from build123d import *

# Parameters (mm, degrees)
F1_DEPTH = 50.8
F3_DEPTH = 25.4
F5_DEPTH = 25.4
F7_DEPTH = 2.54
F8_W     = 5.829871
F8_H     = 7.639144
F9_DEPTH = 2.54


with BuildPart() as f1:
    # F0 (on Front) → F1 (new body)
    with BuildSketch(Plane.XZ):
        Polygon((0, 6.35), (0, 0), (19.05, 0), (19.05, 63.5), (9.525, 63.5), (9.525, 6.35), align=None)
    extrude(amount=F1_DEPTH)

    # F2 (on face) → F3 (cut)
    with BuildSketch(Plane.XY.offset(6.35)):
        with BuildLine():
            ThreePointArc((0, -6.35), (1.859872, -1.859872), (6.35, 0))
            Line((6.35, 0), (0, 0))
            Line((0, 0), (0, -6.35))
        make_face()
        with BuildLine():
            Line((0, -50.8), (6.35, -50.8))
            ThreePointArc((6.35, -50.8), (1.859872, -48.940128), (0, -44.45))
            Line((0, -44.45), (0, -50.8))
        make_face()
    extrude(amount=-F3_DEPTH, mode=Mode.SUBTRACT)

    # F4 (on face) → F5 (cut)
    with BuildSketch(Plane(origin=(9.525, 0, 0), x_dir=(0, -1, 0), z_dir=(-1, 0, 0))):
        with BuildLine():
            ThreePointArc((0, 57.15), (1.859872, 61.640128), (6.35, 63.5))
            Line((6.35, 63.5), (0, 63.5))
            Line((0, 63.5), (0, 57.15))
        make_face()
        with BuildLine():
            ThreePointArc((44.45, 63.5), (48.940128, 61.640128), (50.8, 57.15))
            Line((50.8, 57.15), (50.8, 63.5))
            Line((50.8, 63.5), (44.45, 63.5))
        make_face()
    extrude(amount=-F5_DEPTH, mode=Mode.SUBTRACT)

    # F6 (on face) → F7 (cut)
    with BuildSketch(Plane(origin=(9.525, 0, 0), x_dir=(0, -1, 0), z_dir=(-1, 0, 0))):
        Polygon((6.35, 50.224786), (6.35, 43.83772), (12.7, 43.83772), (12.7, 49.350649), (19.05, 49.350649), (19.05, 39.655992), (12.7, 39.655992), (12.7, 26.955992), (19.05, 26.955992), (19.05, 17.261336), (12.7, 17.261336), (12.7, 20.796465), (6.35, 20.796465), (6.35, 13.726207), (12.7, 10.572023), (19.05, 10.572023), (23.714906, 13.726207), (23.714906, 32.776207), (22.196746, 33.305992), (23.714906, 35.193134), (23.714906, 50.224786), (19.05, 54.197977), (12.7, 54.197977), align=None)
    extrude(amount=-F7_DEPTH, mode=Mode.SUBTRACT)

    # F8 (on face) → F9 (cut)
    with BuildSketch(Plane(origin=(9.525, 0, 0), x_dir=(0, -1, 0), z_dir=(-1, 0, 0))):
        Polygon((28.345251, 40.407062), (34.175124, 37.190579), (40.809121, 37.190579), (40.809121, 17.261336), (34.175124, 17.261336), (34.175124, 23.118468), (28.345251, 23.118468), (28.345251, 13.726207), (30.590052, 10.572023), (44.45, 10.572023), (46.638995, 13.726207), (46.638995, 50.224786), (44.45, 54.197977), (33.974096, 54.197977), (28.345251, 50.257538), align=None)
        with Locations((37.492122, 46.437966)):
            Rectangle(F8_W, F8_H, mode=Mode.SUBTRACT)
    extrude(amount=-F9_DEPTH, mode=Mode.SUBTRACT)


solid = f1.part
CAD build for the part. Positions are in the model's coordinates, mm. A direction names the side the tool comes from. Coordinates: 2 decimals unless noted, no trailing zeros. Write each loop counter-clockwise with the first axis right and the second up, starting at its lowest first coordinate (ties: lowest second). Pieces come first, ordered by that corner, then holes. Notation, with made-up numbers: (-4, 16.25) - (29, 16.25) arc R23 ccw to (29, 48.25) - close; hole circle Ø7 at (72.5, -9). An arc over 180 degrees is marked (long way). Use a Markdown table: item, result. Add a question column.
Item 1: Band-saw the part on C-C, the plane z = 51.5. Give the cut face in (x, y) (3 decimals).
Item 2: Band-saw the part on B-B, the plane z = 25.5. Give the cut face in (x, y) (3 decimals).
Item 3: Band-saw the part on A-A, the plane y = -26.5. Give the cut face in (x, z) (3 decimals).
Item 4: Band-saw the part on D-D, the plane y = -15. Give the cut face in (x, z) (3 decimals), and give its area (3 significant figures).
Item 5: Drill centre lines: L1, parallel to Y at x = 10, z = 25; L2, parallel to Z at x = 10, y = -35; L3, parallel to Y at x = 12, z = 36. Where is each one in solid material? Low to high. Write a range as from..to.
Item 6: Flat gauge pins, fed straight in: pin 1 (6.5 mm diameter, centred on y = -36.5, z = 47, fed in from -X) (3 decimals); pin 2 (3 mm diameter, centred on x = 10.5, y = -17, fed in from -Z). Where does each tip first touch, or does it go through?
Item 7: 3-axis set-ups, long thin cutter, end or side, ignore diameter. For faces 4 (the face through (10.777, -21.35, 12.127)), 5 (the face through (9.525, -25, 35)), 6 (the face through (14, 0, 29)): which of +Z, -Z, +X, -X, +Y, -Y reach the whole face in a straight line?
Item 8: Mould opens along Z. For faces 1 (the face through (11, -10, 20.796)), 2 (the face through (5, -25, 6.35)), 3 (the face through (1.91, -48.99, 3.22)) say: pulls with the +Z half, pulls with the -Z half, needs draft (parallel to the pull), parting line crosses it, or undercut.
Numbers:
| question | item | result |
|---|---|---|
| 1 | outline | (9.525, -50.8) - (19.05, -50.8) - (19.05, 0) - (9.525, 0) - (9.525, -8.388) - (12.065, -8.388) - (12.065, -22.218) - (9.525, -22.218) - (9.525, -30.12) - (12.065, -30.12) - (12.065, -45.936) - (9.525, -45.936) - close |
| 2 | outline | (9.525, -50.8) - (19.05, -50.8) - (19.05, 0) - (9.525, 0) - (9.525, -19.05) - (12.065, -19.05) - (12.065, -23.715) - (9.525, -23.715) - (9.525, -40.809) - (12.065, -40.809) - (12.065, -46.639) - (9.525, -46.639) - close |
| 3 | outline | (0, 0) - (19.05, 0) - (19.05, 63.5) - (9.525, 63.5) - (9.525, 6.35) - (0, 6.35) - close |
| 4 | outline | (0, 0) - (19.05, 0) - (19.05, 63.5) - (9.525, 63.5) - (9.525, 54.198) - (12.065, 54.198) - (12.065, 49.351) - (9.525, 49.351) - (9.525, 39.656) - (12.065, 39.656) - (12.065, 26.956) - (9.525, 26.956) - (9.525, 17.261) - (12.065, 17.261) - (12.065, 10.572) - (9.525, 10.572) - (9.525, 6.35) - (0, 6.35) - close |
| 4 | area | 604 mm2 |
| 5 | L1 | -50.8..-46.64, -40.81..-23.71, -19.05..0 |
| 5 | L2 | 0..10.57, 17.26..37.19, 42.62..50.26, 54.2..63.5 |
| 5 | L3 | -50.8..-46.64, -40.81..-23.71, -12.7..0 |
| 6 | pin 1 | x = 9.525 |
| 6 | pin 2 | z = 0 |
| 7 | face 4 | -X |
| 7 | face 5 | +Z, -X, +Y, -Y |
| 7 | face 6 | +Z, -Z, +X, -X, +Y |
| 8 | face 1 | undercut |
| 8 | face 2 | pulls with the +Z half |
| 8 | face 3 | needs draft |
